Read the model definition and answer for the solid it produces. Units are mm, in the model's axes. Give positions to 0.01 mm unless a question says otherwise; leave off trailing zeros. Order: outer loops, then holes, each group sorted by start corner. A loop starts at its lowest first (then second) coordinate and runs counter-clockwise, first axis right, second up. Notation, with made-up numbers: (-9.5, -13.5) - (41.5, -13.5) arc R21 ccw to (41.5, 12.5) - close; hole circle Ø2 at (8, 84). An arc over 180 degrees is marked (long way). Use a Markdown table: item, result. Add a question column.
1. Consider L1, parallel to X at y = 0.5, z = 9; L2, parallel to X at y = 1.55, z = 120; L3, parallel to Z at x = -120, y = 0.7. Determine where each line is inside the solid, lowest interval first.
2. A cutting plane is placed at D-D on y = 0.95. State how many separate pieces and enclosed holes the cut face has, and give its area (3 significant figures).
3. A cutting plane is placed at A-A on x = 0. Determine the outline of the cut face in (y, z), and give its area (3 significant figures).
4. For a pull along Z with two mould halves and no side action, classify faces 1 (the cylindrical face through (-180.6, 1.5, -40.1)), 2 (the cylindrical face through (19.52, 1.48, 62)), 3 (the flat face through (3, 3, 80)) as released by +Z, released by -Z, zero draft, split by the parting line, or undercut.
5. A cutting plane is placed at B-B on z = -97.5. Determine the outline of the cut face in (x, y), and give its area (3 significant figures).
6. A cutting plane is placed at C-C on z = -34.5. Determine the outline of the cut face in (x, y).
7. Flat-ended cylindrical pins translate along their axes: P1, Ø1.5, axis at y = 1, z = -14.5, coming from the -X side; P2, Ø1, axis at x = -87.5, y = 1, coming from the -Z side; P3, Ø1.5, axis at x = -25.5, y = 1, coming from the -Z side. Find the tip coordinate at first contact, or state that the pin passes through.
```python
from build123d import *

# Parameters (mm, degrees)
SKETCH_1_R      = 185
SKETCH_1_R_2    = 1.5
SKETCH_1_R_3    = 65
EXTRUDE_1_DEPTH = 3


with BuildPart() as part:
    # 草图1 → 凸台-拉伸1 (new body)
    with BuildSketch(Plane(origin=(0, 0, 0), x_dir=(1, 0, 0), z_dir=(0, 1, 0))):
        with Locations(Location((0, 0, 0), (0, 0, 270))):
            Circle(SKETCH_1_R)
        with Locations(Location((120, 120, 0), (0, 0, 270))):
            Circle(SKETCH_1_R_2, mode=Mode.SUBTRACT)
        with Locations(Location((-120, 120, 0), (0, 0, 270))):
            Circle(SKETCH_1_R_2, mode=Mode.SUBTRACT)
        with Locations(Location((-120, -120, 0), (0, 0, 270))):
            Circle(SKETCH_1_R_2, mode=Mode.SUBTRACT)
        with Locations(Location((120, -120, 0), (0, 0, 270))):
            Circle(SKETCH_1_R_2, mode=Mode.SUBTRACT)
        with Locations(Location((0, 0, 0), (0, 0, 270))):
            Circle(SKETCH_1_R_3, mode=Mode.SUBTRACT)
        with Locations(Location((40, 165, 0), (0, 0, 270))):
            Circle(SKETCH_1_R_2, mode=Mode.SUBTRACT)
        with Locations(Location((40, 120, 0), (0, 0, 270))):
            Circle(SKETCH_1_R_2, mode=Mode.SUBTRACT)
        with Locations(Location((-40, 120, 0), (0, 0, 270))):
            Circle(SKETCH_1_R_2, mode=Mode.SUBTRACT)
        with Locations(Location((-40, 165, 0), (0, 0, 270))):
            Circle(SKETCH_1_R_2, mode=Mode.SUBTRACT)
        with Locations(Location((-40, -165, 0), (0, 0, 270))):
            Circle(SKETCH_1_R_2, mode=Mode.SUBTRACT)
        with Locations(Location((-40, -120, 0), (0, 0, 270))):
            Circle(SKETCH_1_R_2, mode=Mode.SUBTRACT)
        with Locations(Location((40, -120, 0), (0, 0, 270))):
            Circle(SKETCH_1_R_2, mode=Mode.SUBTRACT)
        with Locations(Location((40, -165, 0), (0, 0, 270))):
            Circle(SKETCH_1_R_2, mode=Mode.SUBTRACT)
        with Locations(Location((120, 60, 0), (0, 0, 270))):
            Circle(SKETCH_1_R_2, mode=Mode.SUBTRACT)
        with Locations(Location((120, -60, 0), (0, 0, 270))):
            Circle(SKETCH_1_R_2, mode=Mode.SUBTRACT)
        with Locations(Location((-120, -60, 0), (0, 0, 270))):
            Circle(SKETCH_1_R_2, mode=Mode.SUBTRACT)
        with Locations(Location((-120, 60, 0), (0, 0, 270))):
            Circle(SKETCH_1_R_2, mode=Mode.SUBTRACT)
        with BuildLine():
            Line((-137.5, -75), (-137.5, 75))
            ThreePointArc((-137.5, 75), (-142.5, 80), (-147.5, 75))
            Line((-147.5, 75), (-147.5, -75))
            ThreePointArc((-147.5, -75), (-142.5, -80), (-137.5, -75))
        make_face(mode=Mode.SUBTRACT)
        with BuildLine():
            Line((-102.5, -75), (-102.5, 75))
            ThreePointArc((-102.5, 75), (-97.5, 80), (-92.5, 75))
            Line((-92.5, 75), (-92.5, -75))
            ThreePointArc((-92.5, -75), (-97.5, -80), (-102.5, -75))
        make_face(mode=Mode.SUBTRACT)
        with BuildLine():
            Line((-75, -102.5), (75, -102.5))
            ThreePointArc((75, -102.5), (80, -97.5), (75, -92.5))
            Line((75, -92.5), (-75, -92.5))
            ThreePointArc((-75, -92.5), (-80, -97.5), (-75, -102.5))
        make_face(mode=Mode.SUBTRACT)
        with BuildLine():
            Line((-75, -137.5), (75, -137.5))
            ThreePointArc((75, -137.5), (80, -142.5), (75, -147.5))
            Line((75, -147.5), (-75, -147.5))
            ThreePointArc((-75, -147.5), (-80, -142.5), (-75, -137.5))
        make_face(mode=Mode.SUBTRACT)
        with BuildLine():
            Line((137.5, -75), (137.5, 75))
            ThreePointArc((137.5, 75), (142.5, 80), (147.5, 75))
            Line((147.5, 75), (147.5, -75))
            ThreePointArc((147.5, -75), (142.5, -80), (137.5, -75))
        make_face(mode=Mode.SUBTRACT)
        with BuildLine():
            Line((102.5, -75), (102.5, 75))
            ThreePointArc((102.5, 75), (97.5, 80), (92.5, 75))
            Line((92.5, 75), (92.5, -75))
            ThreePointArc((92.5, -75), (97.5, -80), (102.5, -75))
        make_face(mode=Mode.SUBTRACT)
        with BuildLine():
            Line((-75, 102.5), (75, 102.5))
            ThreePointArc((75, 102.5), (80, 97.5), (75, 92.5))
            Line((75, 92.5), (-75, 92.5))
            ThreePointArc((-75, 92.5), (-80, 97.5), (-75, 102.5))
        make_face(mode=Mode.SUBTRACT)
        with BuildLine():
            Line((-75, 137.5), (75, 137.5))
            ThreePointArc((75, 137.5), (80, 142.5), (75, 147.5))
            Line((75, 147.5), (-75, 147.5))
            ThreePointArc((-75, 147.5), (-80, 142.5), (-75, 137.5))
        make_face(mode=Mode.SUBTRACT)
    extrude(amount=EXTRUDE_1_DEPTH)


solid = part.part
```
Output values:
| question | item | result |
|---|---|---|
| 1 | L1 | -184.78 to -147.5, -137.5 to -102.5, -92.5 to -64.37, 64.37 to 92.5, 102.5 to 137.5, 147.5 to 184.78 |
| 1 | L2 | -140.8 to -121.5, -118.5 to -41.5, -38.5 to 38.5, 41.5 to 118.5, 121.5 to 140.8 |
| 1 | L3 | -140.8 to -121.5, -118.5 to -61.5, -58.5 to 58.5, 61.5 to 118.5, 121.5 to 140.8 |
| 2 | separate pieces | 1 |
| 2 | enclosed holes | 25 |
| 2 | area | 81,500 mm² |
| 3 | outline | (0, -185) - (3, -185) - (3, -147.5) - (0, -147.5) - close; (0, -137.5) - (3, -137.5) - (3, -102.5) - (0, -102.5) - close; (0, -92.5) - (3, -92.5) - (3, -65) - (0, -65) - close; (0, 65) - (3, 65) - (3, 92.5) - (0, 92.5) - close; (0, 102.5) - (3, 102.5) - (3, 137.5) - (0, 137.5) - close; (0, 147.5) - (3, 147.5) - (3, 185) - (0, 185) - close |
| 3 | area | 600 mm² |
| 4 | face 1 | split by the parting line |
| 4 | face 2 | undercut |
| 4 | face 3 | zero draft |
| 5 | outline | (-157.22, 0) - (-80, 0) - (-80, 3) - (-157.22, 3) - close; (80, 0) - (157.22, 0) - (157.22, 3) - (80, 3) - close |
| 5 | area | 463 mm² |
| 6 | outline | (-181.75, 0) - (-147.5, 0) - (-147.5, 3) - (-181.75, 3) - close; (-137.5, 0) - (-102.5, 0) - (-102.5, 3) - (-137.5, 3) - close; (-92.5, 0) - (-55.09, 0) - (-55.09, 3) - (-92.5, 3) - close; (55.09, 0) - (92.5, 0) - (92.5, 3) - (55.09, 3) - close; (102.5, 0) - (137.5, 0) - (137.5, 3) - (102.5, 3) - close; (147.5, 0) - (181.75, 0) - (181.75, 3) - (147.5, 3) - close |
| 7 | P1 | x = -184.49 |
| 7 | P2 | z = -163.27 |
| 7 | P3 | z = -183.34 |
